Part model, mm, in its own coordinate system. Face numbers are marked on the shaded views. A direction names the side the tool comes from. Give positions to 0.01 mm unless a question says otherwise; leave off trailing zeros. Write each loop counter-clockwise with the first axis right and the second up, starting at its lowest first coordinate (ties: lowest second). Pieces come first, ordered by that corner, then holes. Notation, with made-up numbers: M 49.25,26 L 70.25,26 A31 ccw 70.25,62 Z; hole C 58.5,59 d3. An arc over 180 degrees is marked long. Answer as CSV lines item,"result". Start each with the question number.
1) Tool access for the marked faces 1, 2, 3 and 4: list every direction of +Z, -Z, +X, -X, +Y, -Y with a clear straight run to the whole face (end or side of a thin tool).
2) Slice it at D-D, the plane z = 5.5. Give the cut face in (x, y).
3) Wall check: line 1 along Z through (x, y) = (1.9, -35); line 2 along X through (y, z) = (-28.5, 2); line 3 along Y through (x, z) = (2.1, 10). Give the ranges that are in metal, low to high. Write a range as from..to.
4) Slice it at B-B, the plane y = -14. Give the number of separate pieces and of enclosed holes in the cut face, plus the area to 3 significant figures.
5) Slice it at A-A, the plane x = 7.5. Give the cut face in (y, z).
6) Slice it at C-C, the plane y = -25. Give the cut face in (x, z) (3 decimals).
7) Pin check, flat tips, straight feed: pin 1 Ø5.5 at (x, z) = (16.5, 1.5) entering from -Y; pin 2 Ø12.5 at (x, y) = (31, -20) entering from +Z; pin 3 Ø1.5 at (y, z) = (-5, 13.5) entering from -X; pin 4 Ø2 at (y, z) = (-21, 10) entering from -X. Stop position of each tip, or through.
8) Mould opens along Y. For the marked faces 5, 6 and 7 say: pulls with the +Y half, pulls with the -Y half, needs draft (parallel to the pull), parting line crosses it, or undercut.
```python
from build123d import *

# Parameters (mm, degrees)
PAD_DEPTH        = 16
POCKET_DEPTH     = 45.001
POCKET001_DEPTH  = 11.001
SKETCH003_R      = 7
PAD001_DEPTH     = 2.5
POCKET002_DEPTH  = 6.9
SKETCH005_R      = 1.6
POCKET003_DEPTH  = 38.001
POCKET004_DEPTH  = 4
CHAMFER_SIZE     = 2
CHAMFER001_SIZE  = 3.79
CHAMFER002_SIZE  = 1.5
CHAMFER003_SIZE2 = 4
CHAMFER003_SIZE  = 0.2
SKETCH007_W      = 0.1
SKETCH007_H      = 3.5
POCKET005_DEPTH  = 21
SKETCH008_W      = 0.1
SKETCH008_H      = 3.5
POCKET006_DEPTH  = 18
SKETCH009_W      = 0.1
SKETCH009_H      = 3.5
POCKET007_DEPTH  = 22
SKETCH010_W      = 0.1
SKETCH010_H      = 3.5
POCKET008_DEPTH  = 20


with BuildPart() as body001:
    # Sketch → Pad (new body)
    with BuildSketch(Plane.XY):
        Polygon((0, 45), (2.2, 45), (8, 39.2), (8, 33), (12.041452, 26), (19.958548, 26), (24, 33), (33, 33), (38, 28), (38, 5), (33, 0), (6, 0), (0, 6), align=None)
        Polygon((20, 21.928203), (12, 21.928203), (8, 15), (12, 8.071797), (20, 8.071797), (24, 15), align=None, mode=Mode.SUBTRACT)
    extrude(amount=PAD_DEPTH)

    # Sketch001 → Pocket (cut, through all)
    with BuildSketch(Plane.XZ):
        Polygon((0, 16), (2, 16), (4, 14), (4, 12), (28.5, 12), (33, 7.5), (33, 5), (39, 5), (39, 17), (0, 17), align=None)
    extrude(amount=-POCKET_DEPTH, mode=Mode.SUBTRACT)

    # Sketch002 → Pocket001 (cut, through all)
    with BuildSketch(Plane.XY.offset(5)):
        Polygon((8, 45), (8, 3.6), (33, 3.6), (33, -1), (39, -1), (39, 45), align=None)
    extrude(amount=POCKET001_DEPTH, mode=Mode.SUBTRACT)

    # Sketch003 → Pad001 (join)
    with BuildSketch(Plane.XY.offset(5)):
        with Locations((29.3, 8)):
            Circle(SKETCH003_R)
    extrude(amount=PAD001_DEPTH)

    # Sketch004 → Pocket002 (cut)
    with BuildSketch(Plane.XY.offset(7.5)):
        with BuildLine():
            ThreePointArc((30.3, 19.4138), (29.3, 30.675), (28.3, 19.4138))
            Line((28.3, 19.4138), (28.3, 11.924602))
            ThreePointArc((28.3, 11.924602), (29.3, 3.95), (30.3, 11.924602))
            Line((30.3, 19.4138), (30.3, 11.924602))
        make_face()
    extrude(amount=-POCKET002_DEPTH, mode=Mode.SUBTRACT)

    # Sketch005 → Pocket003 (cut, through all)
    with BuildSketch(Plane.YZ):
        with Locations((15, 10)):
            Circle(SKETCH005_R)
        with Locations((35, 10)):
            Circle(SKETCH005_R)
    extrude(amount=POCKET003_DEPTH, mode=Mode.SUBTRACT)

    # Sketch006 → Pocket004 (cut)
    with BuildSketch(Plane.YZ.offset(8)):
        with BuildLine():
            ThreePointArc((11.9, 10), (15, 6.9), (18.1, 10))
            Line((18.1, 16), (18.1, 10))
            Line((11.9, 16), (18.1, 16))
            Line((11.9, 10), (11.9, 16))
        make_face()
        with BuildLine():
            ThreePointArc((31.9, 10), (35, 6.9), (38.1, 10))
            Line((38.1, 16), (38.1, 10))
            Line((31.9, 16), (38.1, 16))
            Line((31.9, 10), (31.9, 16))
        make_face()
    extrude(amount=-POCKET004_DEPTH, mode=Mode.SUBTRACT)

    # Chamfer
    chamfer_edges = [body001.edges().sort_by_distance(p)[0] for p in [
        (8, 7.75, 12),
        (8, 25, 12),
        (8, 38.65, 12),
    ]]
    chamfer(chamfer_edges, length=CHAMFER_SIZE)

    # Chamfer001
    chamfer001_edges = [body001.edges().sort_by_distance(p)[0] for p in [
        (1, 45, 16),
    ]]
    chamfer(chamfer001_edges, length=CHAMFER001_SIZE)

    # Chamfer002
    chamfer002_edges = [body001.edges().sort_by_distance(p)[0] for p in [
        (3, 3, 0),
        (19.5, 0, 0),
    ]]
    chamfer(chamfer002_edges, length=CHAMFER002_SIZE)

    # Chamfer003
    chamfer003_edges = [body001.edges().sort_by_distance(p)[0] for p in [
        (29.3, 3.95, 7.5),
    ]]
    chamfer003_side = body001.faces().sort_by_distance((33.19017, 2.828889, 7.5))[0]
    chamfer(chamfer003_edges, length=CHAMFER003_SIZE, length2=CHAMFER003_SIZE2, reference=chamfer003_side)

    # Sketch007 → Pocket005 (cut)
    with BuildSketch(Plane.YZ.offset(1.5)):
        with Locations((24.05, 2.25)):
            Rectangle(SKETCH007_W, SKETCH007_H)
    extrude(amount=POCKET005_DEPTH, mode=Mode.SUBTRACT)

    # Sketch008 → Pocket006 (cut)
    with BuildSketch(Plane.YZ.offset(3)):
        with Locations((6.05, 2.25)):
            Rectangle(SKETCH008_W, SKETCH008_H)
    extrude(amount=POCKET006_DEPTH, mode=Mode.SUBTRACT)

    # Sketch009 → Pocket007 (cut)
    with BuildSketch(Plane.YZ.offset(10)):
        with Locations((2.05, 2.25)):
            Rectangle(SKETCH009_W, SKETCH009_H)
    extrude(amount=POCKET007_DEPTH, mode=Mode.SUBTRACT)

    # Sketch010 → Pocket008 (cut)
    with BuildSketch(Plane.XZ.offset(-6.5)):
        with Locations((36.55, 2.25)):
            Rectangle(SKETCH010_W, SKETCH010_H)
    extrude(amount=-POCKET008_DEPTH, mode=Mode.SUBTRACT)


with BuildPart() as z_axis_top_l:
    # Part__Mirroring: instance of Body001
    add(body001.part.mirror(Plane(origin=(0, 0, 0), x_dir=(1, 0, 0), z_dir=(0, 1, 0))))


solid = z_axis_top_l.part
```
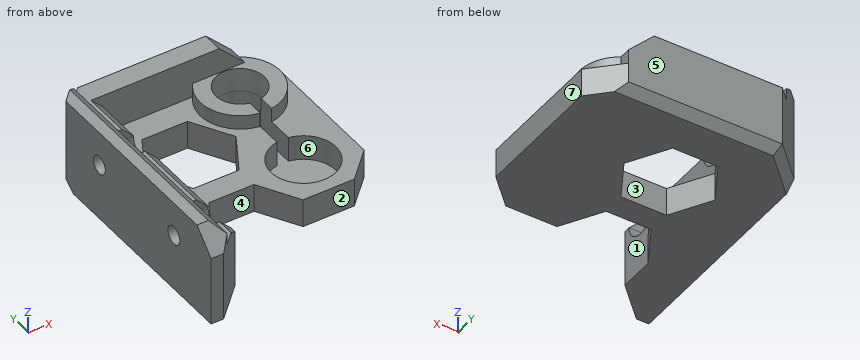
Found:
1,face 1,"+Z, -Y"
1,face 2,"+Z, -Z, +X, -Y"
1,face 3,"+Z, -Z"
1,face 4,"+Z, -Z, -Y"
2,outline,"M 0,-45 L 2.2,-45 L 8,-39.2 L 8,-3.6 L 23.86,-3.6 A7 ccw 28.3,-14.93 L 28.3,-12.03 A4.15 cw long 30.3,-12.03 L 30.3,-14.93 A7 ccw 33,-2.06 L 33,0 L 6,0 L 0,-6 Z"
3,line 1,"0..8.4, 11.6..16"
3,line 2,"0..10.6, 21.4..24.83, 33.77..37.5"
3,line 3,"-45..-36.6, -33.4..-16.6, -13.4..-3.9"
4,separate pieces,"3"
4,enclosed holes,"1"
4,area,"160 mm²"
5,outline,"M -39.7,0 L -1.5,0 L 0,1.5 L 0,12 L -3.6,12 L -3.6,10.5 L -11.9,10.5 L -11.9,10 A3.1 cw -18.1,10 L -18.1,10.5 L -31.9,10.5 L -31.9,10 A3.1 cw -38.1,10 L -38.1,10.5 L -39.7,10.5 Z; hole M -24.1,0.5 L -24,0.5 L -24,4 L -24.1,4 Z; hole M -6.1,0.5 L -6,0.5 L -6,4 L -6.1,4 Z"
6,outline,"M 0,0 L 38,0 L 38,5 L 34.975,5 L 34.975,0.6 L 23.625,0.6 L 23.625,5 L 8,5 L 8,10 L 6,12 L 4,12 L 4,14 L 2,16 L 0,16 Z; hole M 36.5,0.5 L 36.6,0.5 L 36.6,4 L 36.5,4 Z"
7,pin 1,"y = -26"
7,pin 2,"z = 7.5"
7,pin 3,"x = 0.25"
7,pin 4,"x = 0"
8,face 5,"pulls with the +Y half"
8,face 6,"undercut"
8,face 7,"needs draft"
